```python
from build123d import *

# Parameters (mm, degrees)
SKETCH_1_W          = 30
SKETCH_1_H          = 30
EXTRUDE_1_DEPTH     = 3
SKETCH_2_R          = 1.5
CUT_EXTRUDE_1_DEPTH = 3.5
SKETCH_3_W          = 30
SKETCH_3_H          = 3
EXTRUDE_2_DEPTH     = 27
SKETCH_4_R          = 1.5
CUT_EXTRUDE_2_DEPTH = 27
FILLET_1_R          = 1
FILLET_2_R          = 1
SKETCH_5_W          = 30
SKETCH_5_H          = 8
CUT_EXTRUDE_3_DEPTH = 10


with BuildPart() as part:
    # 草图1 → 凸台-拉伸1 (new body)
    with BuildSketch(Plane.XY):
        Rectangle(SKETCH_1_W, SKETCH_1_H)
    extrude(amount=EXTRUDE_1_DEPTH)

    # 草图2 → 切除-拉伸1 (cut)
    with BuildSketch(Plane.XY.offset(3)):
        with Locations((10, 3)):
            Circle(SKETCH_2_R)
        with Locations((-10, 3)):
            Circle(SKETCH_2_R)
    extrude(amount=-CUT_EXTRUDE_1_DEPTH, mode=Mode.SUBTRACT)

    # 草图3 → 凸台-拉伸2 (add)
    with BuildSketch(Plane.XY.offset(3)):
        with Locations((0, -13.5)):
            Rectangle(SKETCH_3_W, SKETCH_3_H)
    extrude(amount=EXTRUDE_2_DEPTH)

    # 草图4 → 切除-拉伸2 (cut)
    with BuildSketch(Plane(origin=(0, -12, 0), x_dir=(1, 0, 0), z_dir=(0, 1, 0))):
        with Locations(Location((10, -18, 0), (0, 0, 270))):
            Circle(SKETCH_4_R)
        with Locations(Location((-10, -18, 0), (0, 0, 270))):
            Circle(SKETCH_4_R)
    extrude(amount=-CUT_EXTRUDE_2_DEPTH, mode=Mode.SUBTRACT)

    # 圆角1
    fillet_1_edges = [part.edges().sort_by_distance(p)[0] for p in [
        (0, -12, 3),
    ]]
    fillet(fillet_1_edges, radius=FILLET_1_R)

    # 圆角2
    fillet_2_edges = [part.edges().sort_by_distance(p)[0] for p in [
        (0, -15, 0),
    ]]
    fillet(fillet_2_edges, radius=FILLET_2_R)

    # 草图5 → 切除-拉伸3 (cut)
    with BuildSketch(Plane(origin=(0, -12, 0), x_dir=(1, 0, 0), z_dir=(0, 1, 0))):
        with Locations((0, -26)):
            Rectangle(SKETCH_5_W, SKETCH_5_H)
    extrude(amount=-CUT_EXTRUDE_3_DEPTH, mode=Mode.SUBTRACT)


solid = part.part
```
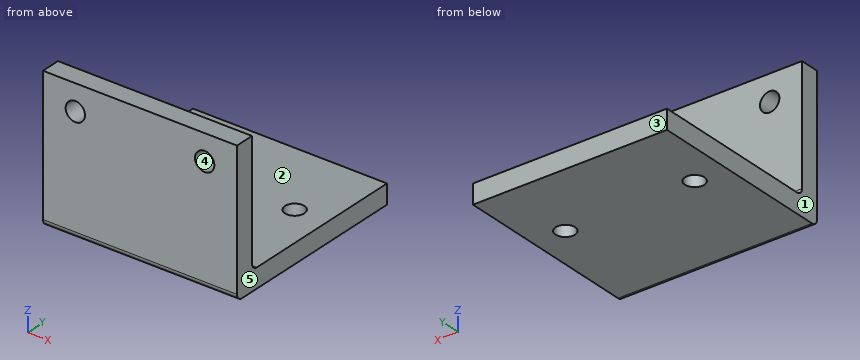
For this review, take the finished solid that the model builds, in its own axes (mm). Face numbers are marked on the shaded views. A direction names the side the tool comes from. Give positions to 0.01 mm unless a question says otherwise; leave off trailing zeros. Order: outer loops, then holes, each group sorted by start corner. A loop starts at its lowest first (then second) coordinate and runs counter-clockwise, first axis right, second up.
1) Wall thickness on line 1 (X direction, y = -14.15, z = 18); line 2 (Y direction, x = 10, z = 2.05); line 3 (Y direction, x = 6.5, z = 14.5): over which ranges is each line inside the solid? List them lowest first.
2) For the marked faces 1 and 2, list the 3-axis set-ups (+Z, -Z, +X, -X, +Y, -Y) from which the entire face can be reached by the end or side of a thin tool; tool diameter is ignored.
3) The part is to be moulded in two halves that separate along X. For the marked faces 3, 4 and 5, say which applies: released by +X, released by -X, zero draft, split by the parting line, or undercut.
4) Insertion check: pin 1 (1 mm diameter, centred on x = 3, z = 16, fed in from +Y); pin 2 (13 mm diameter, centred on x = -1.5, y = 6, fed in from +Z). Each pin has a flat end and moves straight along its axis. Give the tip position at first contact, or say it passes through.
5) Take a section at A-A (y = 3). Give the boundary of the cut face in (x, z), then the cut area to 3 significant figures.
6) Take a section at C-C (x = 10). Give the boundary of the cut face in (y, z).
7) Take a section at B-B (z = 18). Give the boundary of the cut face in (x, y).
8) Take a section at D-D (x = 2). Give the boundary of the cut face in (y, z).
Derived:
1. line 1: x = -15 to -11.5, -8.5 to 8.5, 11.5 to 15
1. line 2: y = -15 to 1.5, 4.5 to 15
1. line 3: y = -15 to -12
2. face 1: +Z, -Z, -X, +Y, -Y
2. face 2: +Z, +X, -X, +Y
3. face 3: zero draft
3. face 4: undercut
3. face 5: released by +X
4. pin 1: stops at y = -12
4. pin 2: stops at z = 3
5. outline: (-15, 0) - (-11.5, 0) - (-11.5, 3) - (-15, 3) - close; (-8.5, 0) - (8.5, 0) - (8.5, 3) - (-8.5, 3) - close; (11.5, 0) - (15, 0) - (15, 3) - (11.5, 3) - close
5. area: 72.0 mm2
6. outline: (-15, 1) arc R1 ccw to (-14, 0) - (1.5, 0) - (1.5, 3) - (-11, 3) arc R1 cw to (-12, 4) - (-12, 16.5) - (-15, 16.5) - close; (-15, 19.5) - (-12, 19.5) - (-12, 22) - (-15, 22) - close; (4.5, 0) - (15, 0) - (15, 3) - (4.5, 3) - close
7. outline: (-15, -15) - (-11.5, -15) - (-11.5, -12) - (-15, -12) - close; (-8.5, -15) - (8.5, -15) - (8.5, -12) - (-8.5, -12) - close; (11.5, -15) - (15, -15) - (15, -12) - (11.5, -12) - close
8. outline: (-15, 1) arc R1 ccw to (-14, 0) - (15, 0) - (15, 3) - (-11, 3) arc R1 cw to (-12, 4) - (-12, 22) - (-15, 22) - close
